Source: CAD feature listing. Evaluate the final solid. Frame: model axes, mm. A direction names the side the tool comes from. Round coordinates to 2 decimals unless told otherwise and drop trailing zeros. Write each loop counter-clockwise with the first axis right and the second up, starting at its lowest first coordinate (ties: lowest second). Pieces come first, ordered by that corner, then holes. Notation, with made-up numbers: M 80,22.5 L 99,22.5 A25 ccw 99,52.5 Z; hole C 76,54.25 d3. An arc over 180 degrees is marked long. Use a Markdown table: item, result.
```python
from build123d import *

# Parameters (mm, degrees)
EXTRUDE_1_DEPTH     = 5
SKETCH_2_R          = 1.75
EXTRUDE_2_DEPTH     = 6
SKETCH_3_W          = 20
SKETCH_3_H          = 5
EXTRUDE_3_DEPTH     = 20
SKETCH_4_R          = 2.5
CUT_EXTRUDE_1_DEPTH = 105.326410846
SKETCH_5_W          = 6
SKETCH_5_H          = 40
EXTRUDE_4_DEPTH     = 10
EXTRUDE_5_DEPTH     = 6
CUT_EXTRUDE_2_REACH = 126.599
SKETCH_8_R          = 1.75
EXTRUDE_6_DEPTH     = 10
CUT_EXTRUDE_3_REACH = 106.109
CUT_EXTRUDE_4_REACH = 117.472
SKETCH_16_W         = 6
SKETCH_16_H         = 6
CUT_EXTRUDE_5_DEPTH = 10
SKETCH_17_W         = 8
SKETCH_17_H         = 5
EXTRUDE_7_DEPTH     = 5


with BuildPart() as part:
    # 草图1 → 凸台-拉伸1 (new body)
    with BuildSketch(Plane(origin=(0, 0, 0), x_dir=(1, 0, 0), z_dir=(0, 1, 0))):
        Polygon((0, 0), (0, 20), (-20, 20), (-20, -16), (100, -16), (100, 0), align=None)
    extrude(amount=EXTRUDE_1_DEPTH)

    # 草图2 → 凸台-拉伸2 (add)
    with BuildSketch(Plane(origin=(100, 0, 0), x_dir=(0, 0, -1), z_dir=(1, 0, 0))):
        Polygon((-16, 0), (-28, 5), (-28, 15), (12, 15), (12, 5), (0, 0), align=None)
        with Locations((-23, 9.2)):
            Circle(SKETCH_2_R, mode=Mode.SUBTRACT)
        with Locations((7, 9.2)):
            Circle(SKETCH_2_R, mode=Mode.SUBTRACT)
    extrude(amount=-EXTRUDE_2_DEPTH)

    # 草图3 → 凸台-拉伸3 (add)
    with BuildSketch(Plane.ZY.offset(20)):
        with Locations((-10, 2.5)):
            Rectangle(SKETCH_3_W, SKETCH_3_H)
    extrude(amount=EXTRUDE_3_DEPTH)

    # 草图4 → 切除-拉伸1 (cut, through all)
    with BuildSketch(Plane(origin=(0, 5, 0), x_dir=(1, 0, 0), z_dir=(0, 1, 0))):
        with Locations(Location((-32.5, 10, 0), (0, 0, 270))):
            Circle(SKETCH_4_R)
        with Locations(Location((-7.5, 10, 0), (0, 0, 270))):
            Circle(SKETCH_4_R)
    extrude(amount=-CUT_EXTRUDE_1_DEPTH, mode=Mode.SUBTRACT)

    # 草图5 → 凸台-拉伸4 (add)
    with BuildSketch(Plane(origin=(0, 5, 0), x_dir=(1, 0, 0), z_dir=(0, 1, 0))):
        with Locations((-17, 10)):
            Rectangle(SKETCH_5_W, SKETCH_5_H)
    extrude(amount=EXTRUDE_4_DEPTH)

    # 草图7 → 凸台-拉伸5 (add)
    with BuildSketch(Plane.ZY.offset(20)):
        Polygon((-30, 5), (-20, 0), (-20, 5), align=None)
    extrude(amount=-EXTRUDE_5_DEPTH)

    # 草图8 → 切除-拉伸2 (cut, up to next)
    with BuildSketch(Plane.ZY.offset(20), mode=Mode.PRIVATE) as cut_extrude_2_sk1:
        with Locations((-25, 9.2)):
            Circle(SKETCH_8_R)
    cut_extrude_2_tool1 = extrude(cut_extrude_2_sk1.sketch, amount=-CUT_EXTRUDE_2_REACH, mode=Mode.PRIVATE) & part.part
    # 草图8 → 切除-拉伸2 (cut, up to next)
    with BuildSketch(Plane.ZY.offset(20), mode=Mode.PRIVATE) as cut_extrude_2_sk2:
        with Locations((5, 9.2)):
            Circle(SKETCH_8_R)
    cut_extrude_2_tool2 = extrude(cut_extrude_2_sk2.sketch, amount=-CUT_EXTRUDE_2_REACH, mode=Mode.PRIVATE) & part.part
    add(cut_extrude_2_tool1.solids().sort_by_distance((-20, 9.2, -25))[0], mode=Mode.SUBTRACT)
    add(cut_extrude_2_tool2.solids().sort_by_distance((-20, 9.2, 5))[0], mode=Mode.SUBTRACT)

    # 草图13 → 凸台-拉伸6 (add)
    with BuildSketch(Plane.ZY.offset(-94)):
        Polygon((-12, 5), (28, 5), (16, 0), (0, 0), align=None)
    extrude(amount=EXTRUDE_6_DEPTH)

    # 草图14 → 切除-拉伸3 (cut, up to next)
    with BuildSketch(Plane(origin=(41.704918033, 0, -34.754098361), x_dir=(-0.6401843996644796, 0, -0.7682212795973761), z_dir=(0.7682212795973761, 0, -0.6401843996644796)), mode=Mode.PRIVATE) as cut_extrude_3_sk1:
        Polygon((-66.067030045, 5), (-66.067030045, 0), (-81.687529397, 5), align=None)
    cut_extrude_3_tool1 = extrude(cut_extrude_3_sk1.sketch, amount=-CUT_EXTRUDE_3_REACH, mode=Mode.PRIVATE) & part.part
    add(cut_extrude_3_tool1.solids().sort_by_distance((87.333333, 3.333333, 20))[0], mode=Mode.SUBTRACT)

    # 草图15 → 切除-拉伸4 (cut, up to next)
    with BuildSketch(Plane(origin=(49.573770492, 0, 41.31147541), x_dir=(0.6401843996644798, 0, -0.768221279597376), z_dir=(0.768221279597376, 0, 0.6401843996644798)), mode=Mode.PRIVATE) as cut_extrude_4_sk1:
        Polygon((69.395988924, 5), (53.775489572, 0), (53.775489572, 5), align=None)
    cut_extrude_4_tool1 = extrude(cut_extrude_4_sk1.sketch, amount=-CUT_EXTRUDE_4_REACH, mode=Mode.PRIVATE) & part.part
    add(cut_extrude_4_tool1.solids().sort_by_distance((87.333333, 3.333333, -4))[0], mode=Mode.SUBTRACT)

    # 草图16 → 切除-拉伸5 (cut)
    with BuildSketch(Plane(origin=(0, 5, 0), x_dir=(1, 0, 0), z_dir=(0, 1, 0))):
        with Locations((-17, -13)):
            Rectangle(SKETCH_16_W, SKETCH_16_H)
    extrude(amount=-CUT_EXTRUDE_5_DEPTH, mode=Mode.SUBTRACT)

    # 草图17 → 凸台-拉伸7 (add)
    with BuildSketch(Plane(origin=(0, 0, 0), x_dir=(-1, 0, 0), z_dir=(0, 0, -1))):
        with Locations((-4, 2.5)):
            Rectangle(SKETCH_17_W, SKETCH_17_H)
    extrude(amount=EXTRUDE_7_DEPTH)


solid = part.part
```
Q1. Section C-C on y = 3.5. Return loops of the section in (x, z).
Results are:
| item | result |
|---|---|
| outline | M -40,-20 L -20,-20 L -20,-27 L -14,-27 L -14,-20 L 0,-20 L 0,-5 L 8,-5 L 8,0 L 84,0 L 91,-8.4 L 100,-8.4 L 100,24.4 L 91,24.4 L 84,16 L -14,16 L -14,10 L -20,10 L -20,0 L -40,0 Z; hole C -32.5,-10 d5; hole C -7.5,-10 d5 |
Q2. First-contact query: pin 1 Ø4 at (x, y) = (-3.5, 1.5) entering from -Z; pin 2 Ø2 at (y, z) = (9.2, -7) entering from +X; pin 3 Ø1 at (x, y) = (71, 3.5) entering from +Z; pin 4 Ø3 at (y, z) = (9.2, 23) entering from -X. Flat tips, straight axial feed; report the tip coordinate or a pass-through.
Results are:
| item | result |
|---|---|
| pin 1 | z = -20 |
| pin 2 | x = -14 |
| pin 3 | z = 16 |
| pin 4 | through |
Q3. Line query: L1, parallel to X at y = 3.65, z = -10; L2, parallel to X at y = 10.5, z = -10; L3, parallel to X at y = 8, z = 21. Output: solid intervals per line, ascending.
Results are:
| item | result |
|---|---|
| L1 | -40 to -35, -30 to -10, -5 to 0 |
| L2 | -20 to -14, 94 to 100 |
| L3 | 94 to 100 |
Q4. Section A-A on z = 5. Return loops of the section in (x, y), plus the area to 3 significant figures.
Results are:
| item | result |
|---|---|
| outline | M -20,0 L 100,0 L 100,15 L 94,15 L 94,5 L -14,5 L -14,7.45 L -20,7.45 Z; M -20,10.95 L -14,10.95 L -14,15 L -20,15 Z |
| area | 699 mm^2 |
Q5. Reachability of faces 1 (the flat face through (-30, 2, 0)), 2 (the cylindrical face through (97.042, 9.726, -8.669)), 3 (the flat face through (4, 3, -5)), 4 (the flat face through (97, 10, -12)) from +Z, -Z, +X, -X, +Y, -Y: full face, straight path, thin tool, end or side. Return the list, or none.
Results are:
| item | result |
|---|---|
| face 1 | +Z, -X, +Y, -Y |
| face 2 | +X |
| face 3 | -Z, +Y, -Y |
| face 4 | -Z, +X, +Y, -Y |
Q6. Section D-D on y = 9.2. Return loops of the section in (x, z), plus the area to 3 significant figures.
Results are:
| item | result |
|---|---|
| outline | M -20,-30 L -14,-30 L -14,-26.75 L -20,-26.75 Z; M -20,-23.25 L -14,-23.25 L -14,3.25 L -20,3.25 Z; M -20,6.75 L -14,6.75 L -14,10 L -20,10 Z; M 94,-12 L 100,-12 L 100,-8.75 L 94,-8.75 Z; M 94,-5.25 L 100,-5.25 L 100,21.25 L 94,21.25 Z; M 94,24.75 L 100,24.75 L 100,28 L 94,28 Z |
| area | 396 mm^2 |
Q7. Section B-B on x = -32.5. Return loops of the section in (y, z), plus the area to 3 significant figures.
Results are:
| item | result |
|---|---|
| outline | M 0,-20 L 5,-20 L 5,-12.5 L 0,-12.5 Z; M 0,-7.5 L 5,-7.5 L 5,0 L 0,0 Z |
| area | 75.0 mm^2 |
Q8. Mould query, pull axis X, two halves, no side actions, for faces 5 (the flat face through (-40, 3, -10)), 6 (the flat face through (41, 5, 10)), 7 (the flat face through (-7, 2, -20)). Classes: +X half, -X half, draft (parallel to the pull), parting line (faces both ways), or undercut.
Results are:
| item | result |
|---|---|
| face 5 | -X half |
| face 6 | undercut |
| face 7 | draft |
